Work out the finished part from the listing and answer in its coordinate system (mm). Face numbers are marked on the shaded views. A direction names the side the tool comes from. Give positions to 0.01 mm unless a question says otherwise; leave off trailing zeros.
```python
from build123d import *

# Parameters (mm, degrees)
PAD_DEPTH          = 35
SKETCH003_R        = 4.75
POCKET_DEPTH       = 12.893309
PAD001_DEPTH       = 35
SKETCH005_R        = 8
POCKET001_DEPTH    = 13
POCKET002_DEPTH    = 143.950619
POLARPATTERN_COUNT = 55
FILLET_R           = 4


with BuildPart() as part:
    # Sketch → Pad (new body)
    with BuildSketch(Plane.XY):
        with BuildLine():
            ThreePointArc((15.5, 22.107691), (0, 27), (-15.5, 22.107691))
            Line((-15.5, 22.107691), (-15, 35))
            Line((-15, 35), (15, 35))
            Line((15, 35), (15.5, 22.107691))
        make_face()
    extrude(amount=PAD_DEPTH)

    # Sketch003 (on Face3 of Pad) → Pocket (cut, through all)
    with BuildSketch(Plane(origin=(0, 35, 0), x_dir=(-1, 0, 0), z_dir=(0, 1, 0))):
        with Locations((0, 17.5)):
            Circle(SKETCH003_R)
    extrude(amount=-POCKET_DEPTH, mode=Mode.SUBTRACT)

    # Sketch004 (on Face3 of Pocket) → Pad001 (join)
    with BuildSketch(Plane(origin=(0, 0, 0), x_dir=(1, 0, 0), z_dir=(0, 0, -1))):
        Polygon((-15, -35), (-10.519122, -50.063099), (13.624797, -42.880915), (15, -35), align=None)
    extrude(amount=-PAD001_DEPTH)

    # Sketch005 (on Face12 of Pad001) → Pocket001 (cut)
    with BuildSketch(Plane(origin=(12.826585, 43.118362, 0), x_dir=(-0.95849, 0.285126, 0), z_dir=(0.285126, 0.95849, 0))):
        with Locations((12.213826, 17.5)):
            Circle(SKETCH005_R)
    extrude(amount=-POCKET001_DEPTH, mode=Mode.SUBTRACT)

    # Sketch001 (on Face4 of Pocket001) → Pocket002 (cut, through all)
    with BuildSketch(Plane.XY.offset(35)):
        Polygon((-7.025, 17.032343), (0, 29.2), (7.025, 17.032343), align=None)
    pocket002 = extrude(amount=-POCKET002_DEPTH, mode=Mode.SUBTRACT)

    # PolarPattern: Pocket002 ×55 about axis
    polarpattern_axis = Axis((0, 0, 35), (0, 0, 1))
    for i in range(1, POLARPATTERN_COUNT):
        add(pocket002.rotate(polarpattern_axis, i * 360 / POLARPATTERN_COUNT), mode=Mode.SUBTRACT)

    # Fillet
    fillet_edges = [part.edges().sort_by_distance(p)[0] for p in [
        (13.624797, 42.880915, 17.5),
        (-10.519122, 50.063099, 17.5),
    ]]
    fillet(fillet_edges, radius=FILLET_R)


solid = part.part
```
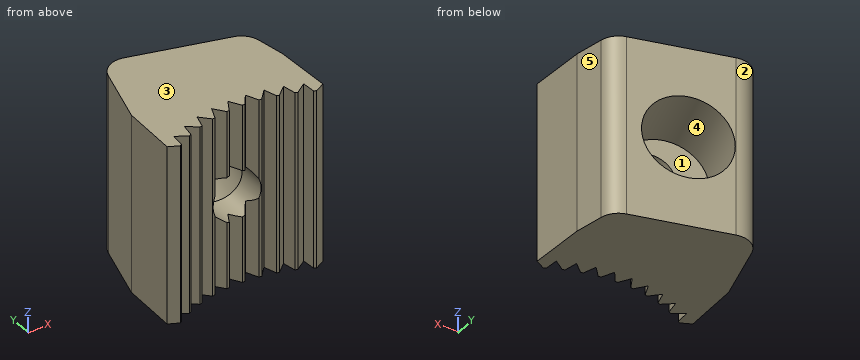
Q1. Which of the six approach directions +Z, -Z, +X, -X, +Y, -Y give full straight-line access (tool end or side, diameter ignored) to the marked faces 1 and 2?
Q2. Consider line 1 along Z through (x, y) = (0, 32); line 2 along Z through (x, y) = (-2.5, 34.75); line 3 along X through (y, z) = (26.75, 29). Determine where each line is inside the solid, lowest interval first.
Q3. Section A-A on y = 28 is taken. State how many separate pieces and enclosed holes the cut face has, plus the area to 3 significant figures.
Q4. Given pin 1 (12 mm diameter, centred on y = 42, z = 26.5, fed in from -X); pin 2 (1.5 mm diameter, centred on x = -11.5, y = 45, fed in from -Z); pin 3 (3 mm diameter, centred on y = 29, z = 20, fed in from +X); pin 4 (2 mm diameter, centred on x = -3.5, z = 31, fed in from +Y), each flat-ended and moving along its own axis, determine where each tip first touches the part or whether it passes through.
Q5. Determine the mould class of the marked faces 3, 4 and 5 for opening direction Y: +Y half, -Y half, draft (parallel to the pull), parting line (faces both ways), or undercut.
Check result:
1. face 1: none
1. face 2: +Z, -Z, +Y
2. line 1: z = 0 to 12.75, 22.25 to 35
2. line 2: z = 0 to 9.5, 25.5 to 35
2. line 3: x = -15.32 to -9.95, -8.93 to -7.13, -5.03 to -4.31, 4.31 to 5.03, 7.13 to 8.93, 9.95 to 15.32
3. separate pieces: 8
3. enclosed holes: 0
3. area: 858 mm2
4. pin 1: stops at x = -14.7
4. pin 2: stops at z = 0
4. pin 3: stops at x = 15.29
4. pin 4: stops at y = 48.27
5. face 3: draft
5. face 4: undercut
5. face 5: +Y half
